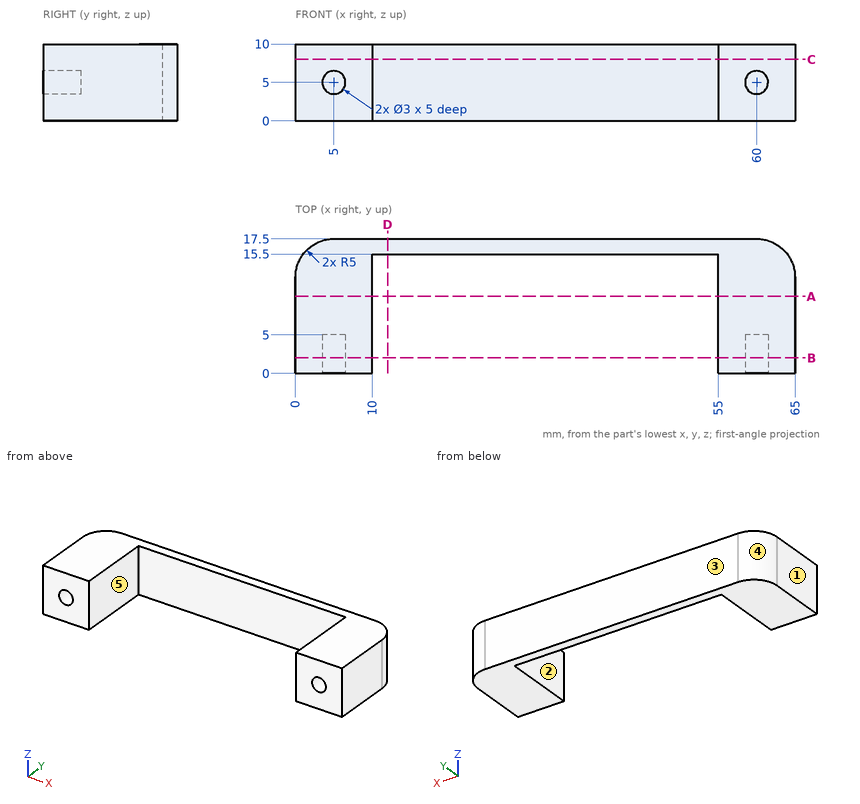
Geometry check sheet. Reference: drawing and pictorial views, mm from the part's lowest x, y, z. A direction names the side the tool comes from. Round coordinates to 2 decimals unless told otherwise and drop trailing zeros. Write each loop counter-clockwise with the first axis right and the second up, starting at its lowest first coordinate (ties: lowest second). Pieces come first, ordered by that corner, then holes.
1. Section check D-D on x = 12. Enter the section's corners in (y, z), plus the area to 3 significant figures.
2. Section check C-C on z = 8. Enter the section's corners in (x, y).
3. Scan lines: L1, parallel to X at y = 3.55, z = 5; L2, parallel to X at y = 12.5, z = 9.5; L3, parallel to Y at x = 19.5, z = 7. Record each from-to range of solid material in increasing order.
4. Access from +Z, -Z, +X, -X, +Y, -Y to the whole of each face (thin tool, end or side, straight path). Record for the marked faces 4 and 5.
5. Draft check along X on the marked faces 1, 2 and 3. Enter one of: +X half, -X half, draft (parallel to the pull), parting line (faces both ways), or undercut.
6. Gauge pin test, flat end, axial feed: P1, Ø1.5, axis at x = 60, z = 5, coming from the -Y side. Record the tip position at first contact, or that the pin passes through.
7. Section check A-A on y = 10. Enter the section's corners in (x, z), plus the area to 3 significant figures.
8. Section check B-B on y = 2. Enter the section's corners in (x, z).
Answer:
1. outline: (15.5, 0) - (17.5, 0) - (17.5, 10) - (15.5, 10) - close
1. area: 20.0 mm2
2. outline: (0, 0) - (10, 0) - (10, 15.5) - (55, 15.5) - (55, 0) - (65, 0) - (65, 12.5) arc R5 ccw to (60, 17.5) - (5, 17.5) arc R5 ccw to (0, 12.5) - close
3. L1: x = 0 to 3.5, 6.5 to 10, 55 to 58.5, 61.5 to 65
3. L2: x = 0 to 10, 55 to 65
3. L3: y = 15.5 to 17.5
4. face 4: +Z, -Z, -X, +Y
4. face 5: +Z, -Z, -Y
5. face 1: -X half
5. face 2: undercut
5. face 3: draft
6. P1: stops at y = 5
7. outline: (0, 0) - (10, 0) - (10, 10) - (0, 10) - close; (55, 0) - (65, 0) - (65, 10) - (55, 10) - close
7. area: 200 mm2
8. outline: (0, 0) - (10, 0) - (10, 10) - (0, 10) - close; (55, 0) - (65, 0) - (65, 10) - (55, 10) - close; hole circle Ø3 at (5, 5); hole circle Ø3 at (60, 5)
